```python
from build123d import *

# Parameters (mm, degrees)
SKETCH1_R           = 77.5
BOSS_EXTRUDE1_DEPTH = 43
SKETCH3_R           = 71
CUT_EXTRUDE1_DEPTH  = 44
SKETCH4_R           = 71
SKETCH4_R_2         = 68.044293834
BOSS_EXTRUDE3_DEPTH = 21


with BuildPart() as part:
    # Sketch1 → Boss-Extrude1 (new body)
    with BuildSketch(Plane(origin=(0, 0, 0), x_dir=(1, 0, 0), z_dir=(0, 1, 0))):
        Circle(SKETCH1_R)
    extrude(amount=BOSS_EXTRUDE1_DEPTH)

    # Sketch3 → Cut-Extrude1 (cut, through all)
    with BuildSketch(Plane.XZ):
        Circle(SKETCH3_R)
    extrude(amount=-CUT_EXTRUDE1_DEPTH, mode=Mode.SUBTRACT)

    # Sketch4 → Boss-Extrude3 (add, through all)
    with BuildSketch(Plane(origin=(0, 22, 0), x_dir=(1, 0, 0), z_dir=(0, 1, 0))):
        Circle(SKETCH4_R)
        Circle(SKETCH4_R_2, mode=Mode.SUBTRACT)
    extrude(amount=BOSS_EXTRUDE3_DEPTH)


solid = part.part
```
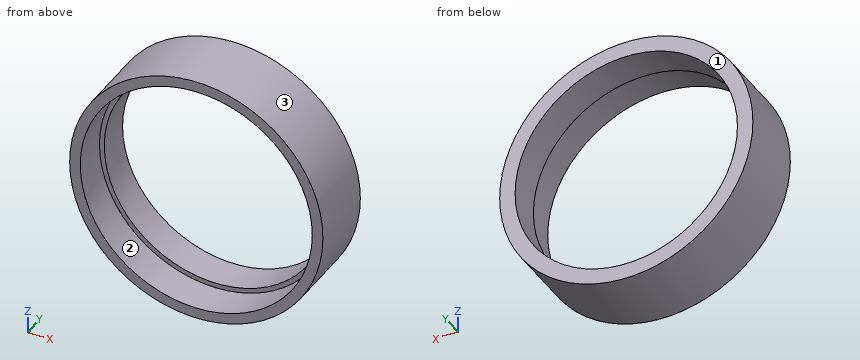
Verification items for the finished model (mm, model axes). Face numbers are marked on the shaded views. Round coordinates to 2 decimals unless told otherwise and drop trailing zeros. Order: outer loops, then holes, each group sorted by start corner. A loop starts at its lowest first (then second) coordinate and runs counter-clockwise, first axis right, second up. Notation, with made-up numbers: (36, 2.25) -> (74, 2.25) arc R30 cw to (74, 24.25) -> close; hole circle Ø7 at (35, -4). An arc over 180 degrees is marked (long way). Put each result on its own line as item: value. Start each with the question number.
(1) Material ranges on line 1 along X through (y, z) = (10.5, 0); line 2 along Z through (x, y) = (0, 31); line 3 along X through (y, z) = (35.5, -1.5), recorded low to high.
(2) Section check C-C (y = 25.5). Enter the section's corners in (x, z), then the cut area to 3 significant figures.
(3) Draft check along X on the marked faces 1, 2 and 3. Enter one of: +X half, -X half, draft (parallel to the pull), parting line (faces both ways), or undercut.
(4) Depth check by flat-ended pin: pin 1 Ø1 at (y, z) = (18.5, -13) entering from -X; pin 2 Ø8 at (y, z) = (4.5, -30) entering from +X; pin 3 Ø1 at (x, y) = (0, 8) entering from +Z. Enter the tip coordinate at first touch or a pass-through.
(5) Section check A-A (x = 0). Enter the section's corners in (y, z).
(6) Section check B-B (z = 0). Enter the section's corners in (x, y).
(7) Section check D-D (y = 7.5). Enter the section's corners in (x, z), then the cut area to 3 significant figures.
Completed:
1. line 1: x = -77.5 to -71, 71 to 77.5
1. line 2: z = -77.5 to -68.04, 68.04 to 77.5
1. line 3: x = -77.49 to -68.03, 68.03 to 77.49
2. outline: circle Ø155 at (0, 0); hole circle Ø136.09 at (0, 0)
2. area: 4,320 mm2
3. face 1: draft
3. face 2: undercut
3. face 3: parting line
4. pin 1: stops at x = -76.49
4. pin 2: stops at x = 73.01
4. pin 3: stops at z = 77.5
5. outline: (0, -77.5) -> (43, -77.5) -> (43, -68.04) -> (22, -68.04) -> (22, -71) -> (0, -71) -> close; (0, 71) -> (22, 71) -> (22, 68.04) -> (43, 68.04) -> (43, 77.5) -> (0, 77.5) -> close
6. outline: (-77.5, 0) -> (-71, 0) -> (-71, 22) -> (-68.04, 22) -> (-68.04, 43) -> (-77.5, 43) -> close; (68.04, 22) -> (71, 22) -> (71, 0) -> (77.5, 0) -> (77.5, 43) -> (68.04, 43) -> close
7. outline: circle Ø155 at (0, 0); hole circle Ø142 at (0, 0)
7. area: 3,030 mm2
